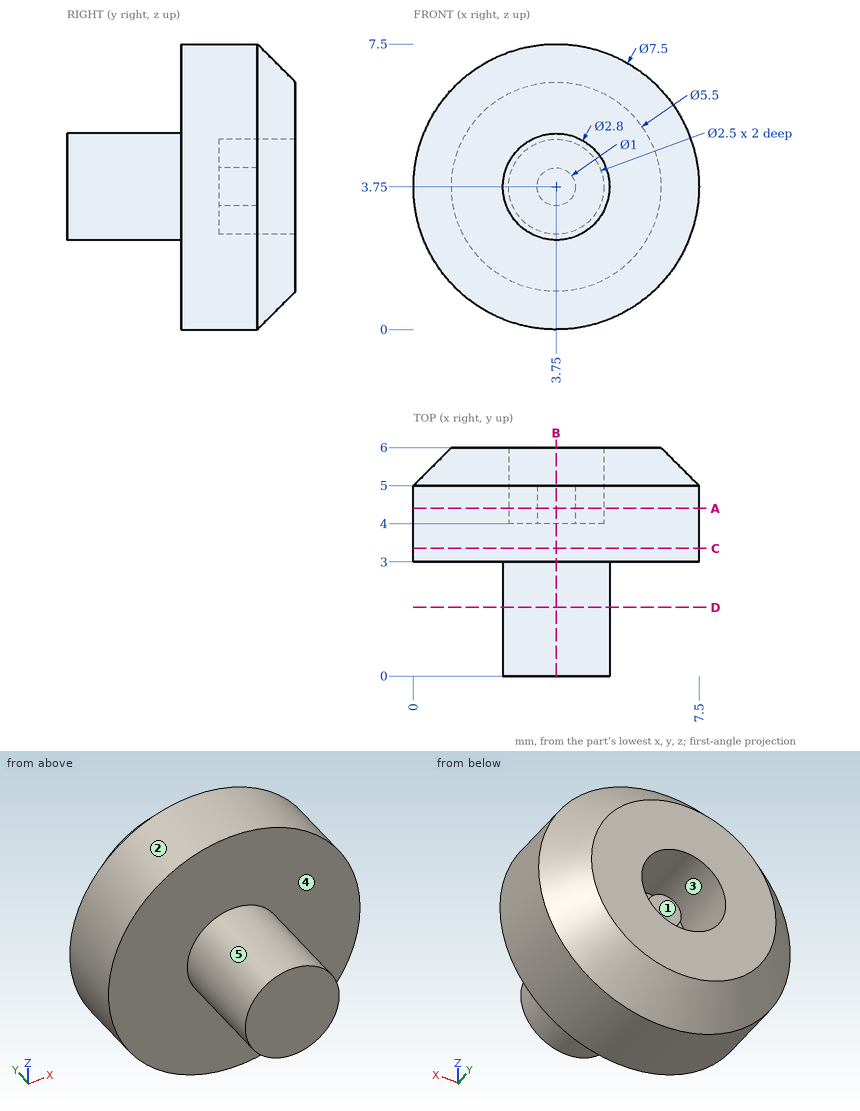
Study the drawing (mm; zero at the part's minimum x, y, z) and answer. A direction names the side the tool comes from. Coordinates: 2 decimals unless noted, no trailing zeros. Write each loop counter-clockwise with the first axis right and the second up, starting at its lowest first coordinate (ties: lowest second). Pieces come first, ordered by that corner, then holes. Notation, with made-up numbers: M 20,81 L 55,81 A9 cw 55,89 Z; hole C 41.5,82 d2. An arc over 180 degrees is marked long. Use one line per item in the form item = value.
Item 1: Find section D-D, the plane y = 1.8. Give the vertices of the cut face in (x, z), plus the area to 3 significant figures.
Model answer:
outline = C 3.75,3.75 d2.8
area = 6.16 mm2
Item 2: Given P1, Ø1.2, axis at x = 4, z = 3.5, coming from the +Y side; P2, Ø4, axis at x = 1.5, z = 1.5, coming from the -Y side; P3, Ø2, axis at x = 3.5, y = 1, coming from the -Z side; P4, Ø1, axis at x = 6.5, z = 6, coming from the +Y side, each flat-ended and moving along its own axis, determine where each tip first touches the part or whether it passes through.
Model answer:
P1 = 5
P2 = 0
P3 = 2.35
P4 = 5.7
Item 3: The mould has two halves that part along Z. Classify the marked faces 3, 4 and 5: released by +Z, released by -Z, zero draft, split by the parting line, or undercut.
Model answer:
face_3 = undercut
face_4 = zero draft
face_5 = split by the parting line
Item 4: For the marked faces 1 and 2, determine the directions among +Z, -Z, +X, -X, +Y, -Y from which every point of the face is accessible in a straight line to the end or side of a thin tool.
Model answer:
face_1 = +Y
face_2 = +Y, -Y
Item 5: Find the intervals of material crossed by probe 1 along X at (y, z) = (4.7, 3.75); probe 2 along Y at (x, z) = (4.5, 3), in increasing order.
Model answer:
probe_1 = 0 to 2.5, 3.25 to 4.25, 5 to 7.5
probe_2 = 0 to 4
Item 6: Find section B-B, the plane x = 3.75. Give the vertices of the cut face in (y, z).
Model answer:
outline = M 0,2.35 L 3,2.35 L 3,0 L 5,0 L 6,1 L 6,2.5 L 4,2.5 L 4,3.25 L 5,3.25 L 5,4.25 L 4,4.25 L 4,5 L 6,5 L 6,6.5 L 5,7.5 L 3,7.5 L 3,5.15 L 0,5.15 Z
Item 7: Find section C-C, the plane y = 3.35. Give the vertices of the cut face in (x, z), plus the area to 3 significant figures.
Model answer:
outline = C 3.75,3.75 d7.5
area = 44.2 mm2
Item 8: Find section A-A, the plane y = 4.4. Give the vertices of the cut face in (x, z).
Model answer:
outline = C 3.75,3.75 d7.5; C 3.75,3.75 d1; hole C 3.75,3.75 d2.5
